Part model, mm, in its own coordinate system. A direction names the side the tool comes from. Give positions to 0.01 mm unless a question says otherwise; leave off trailing zeros. Loops run counter-clockwise (first coordinate to the right, second up) from the corner with the lowest first, then second, coordinate; pieces in that order, holes last. Notation, with made-up numbers: M 12.25,14.5 L 26.25,14.5 A24 cw 26.25,36.5 Z; hole C 46.25,11.5 d11. An arc over 180 degrees is marked long. Answer in a Markdown table with one row per item.
from build123d import *

# Parameters (mm, degrees)
BOSS_EXTRUDE1_DEPTH = 84.85
SKETCH2_R           = 2.1
CUT_EXTRUDE1_DEPTH  = 88.746923023


with BuildPart() as part:
    # Sketch1 → Boss-Extrude1 (new body)
    with BuildSketch(Plane(origin=(0, 0, 0), x_dir=(0, 0, -1), z_dir=(1, 0, 0))):
        Polygon((-10, 20), (-4.900000095, 20), (-3.099999905, 18.200000763), (-5.499340057, 18.200000763), (-5.499340057, 16.559999466), (-2.502582312, 13.590000153), (2.52933979, 13.590000153), (5.499340057, 16.559999466), (5.499340057, 18.200000763), (3.099999905, 18.200000763), (4.900000095, 20), (10, 20), (10, 14.899999619), (8.199999809, 13.100000381), (8.199999809, 15.499340057), (6.559999943, 15.499340057), (3.589999914, 12.52933979), (3.589999914, 7.47066021), (6.559999943, 4.500659943), (8.199999809, 4.500659943), (8.199999809, 6.900000095), (10, 5.099999905), (10, 0), (4.900000095, 0), (3.099999905, 1.799999952), (5.499340057, 1.799999952), (5.499340057, 3.440000057), (2.52933979, 6.409999847), (-2.555858612, 6.409999847), (-5.499340057, 3.440000057), (-5.499340057, 1.799999952), (-3.099999905, 1.799999952), (-4.900000095, 0), (-10, 0), (-10, 5.099999905), (-8.199999809, 6.899999951), (-8.199999809, 4.500659943), (-6.559999943, 4.500659943), (-3.589999914, 7.444141388), (-3.589999914, 12.50258255), (-6.559999943, 15.499340057), (-8.199999809, 15.499340057), (-8.199999809, 13.100000381), (-10, 14.899999619), align=None)
    extrude(amount=BOSS_EXTRUDE1_DEPTH)

    # Sketch2 → Cut-Extrude1 (cut, through all)
    with BuildSketch(Plane(origin=(84.85, 0, 0), x_dir=(0, 0, -1), z_dir=(1, 0, 0))):
        with Locations((5.9664e-05, 10)):
            Circle(SKETCH2_R)
    extrude(amount=-CUT_EXTRUDE1_DEPTH, mode=Mode.SUBTRACT)


solid = part.part
(1) Saw through at A-A (y = 10). Write the cut outline in (x, z), plus the area to 3 significant figures.
Recorded:
| item | result |
|---|---|
| outline | M 0,-3.59 L 84.85,-3.59 L 84.85,-2.1 L 0,-2.1 Z; M 0,2.1 L 84.85,2.1 L 84.85,3.59 L 0,3.59 Z |
| area | 253 mm^2 |
(2) Drill centre lines: line 1 along Z through (x, y) = (5, 9.75) (3 decimals); line 2 along Y through (x, z) = (66, -8); line 3 along Z through (x, y) = (39.5, 6.5). Where is each one in solid material? Low to high.
Recorded:
| item | result |
|---|---|
| line 1 | z = -3.59 to -2.085, 2.085 to 3.59 |
| line 2 | y = 0 to 4.5, 15.5 to 20 |
| line 3 | z = -8.6 to -8.2, -4.56 to 4.54, 8.2 to 8.6 |
(3) Pin check, flat tips, straight feed: pin 1 Ø4 at (x, y) = (38.5, 12) entering from -Z; pin 2 Ø5 at (x, z) = (46.5, 2.5) entering from +Y; pin 3 Ø5 at (x, y) = (74, 10.5) entering from +Z; pin 4 Ø1 at (x, z) = (64.5, 3.5) entering from +Y. Stop position of each tip, or through.
Recorded:
| item | result |
|---|---|
| pin 1 | stops at z = -9.1 |
| pin 2 | stops at y = 20 |
| pin 3 | stops at z = 4.08 |
| pin 4 | stops at y = 19.1 |
(4) Pull direction Y, two halves, no side cores. Call faces 4 (the face through (42, 17, 10)), 5 (the face through (41.831, 4.946, 4.007)), 6 (the face through (41.8, 19.1, 4)): +Y half, -Y half, draft (parallel to the pull), parting line (faces both ways), or undercut.
Recorded:
| item | result |
|---|---|
| face 4 | draft |
| face 5 | undercut |
| face 6 | +Y half |
(5) Which spindle directions (+Z, -Z, +X, -X, +Y, -Y) get a long thin tool onto all of the face, cutting with end or side? Do faces 1 (the face through (41.83, 6.01, -5.05)), 2 (the face through (84.85, 12.4, -0.1)), 3 (the face through (41.8, 0.9, -4)). Say none if no direction does.
Recorded:
| item | result |
|---|---|
| face 1 | +X, -X |
| face 2 | +Z, -Z, +X, +Y, -Y |
| face 3 | +X, -X, -Y |
